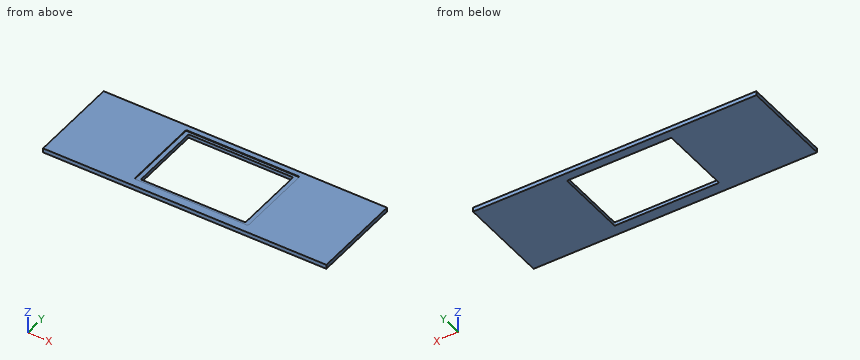
```python
from build123d import *

# Parameters (mm, degrees)
F0_W     = 1990
F0_H     = 645
F1_DEPTH = 30
F3_DEPTH = 5


with BuildPart() as f1:
    # F0 (on Top) → F1 (new body)
    with BuildSketch(Plane.XY):
        with Locations((-995, 322.5)):
            Rectangle(F0_W, F0_H)
        with BuildLine():
            ThreePointArc((-1353.5, 579), (-1351.742641, 583.242641), (-1347.5, 585))
            Line((-1347.5, 585), (-625.5, 585))
            ThreePointArc((-625.5, 585), (-621.257359, 583.242641), (-619.5, 579))
            Line((-619.5, 579), (-619.5, 83))
            ThreePointArc((-619.5, 83), (-621.257359, 78.757359), (-625.5, 77))
            Line((-625.5, 77), (-1347.5, 77))
            ThreePointArc((-1347.5, 77), (-1351.742641, 78.757359), (-1353.5, 83))
            Line((-1353.5, 83), (-1353.5, 579))
        make_face(mode=Mode.SUBTRACT)
    extrude(amount=F1_DEPTH)

    # F2 (on face) → F3 (cut)
    with BuildSketch(Plane.XY.offset(30)):
        with BuildLine():
            Line((-587.5, 65), (-587.5, 597))
            ThreePointArc((-587.5, 597), (-590.136039, 603.363961), (-596.5, 606))
            Line((-596.5, 606), (-1376.5, 606))
            ThreePointArc((-1376.5, 606), (-1382.863961, 603.363961), (-1385.5, 597))
            Line((-1385.5, 597), (-1385.5, 65))
            ThreePointArc((-1385.5, 65), (-1382.863961, 58.636039), (-1376.5, 56))
            Line((-1376.5, 56), (-596.5, 56))
            ThreePointArc((-596.5, 56), (-590.136039, 58.636039), (-587.5, 65))
        make_face()
        with BuildLine():
            Line((-625.5, 77), (-1347.5, 77))
            ThreePointArc((-1347.5, 77), (-1351.742641, 78.757359), (-1353.5, 83))
            Line((-1353.5, 83), (-1353.5, 579))
            ThreePointArc((-1353.5, 579), (-1351.742641, 583.242641), (-1347.5, 585))
            Line((-1347.5, 585), (-625.5, 585))
            ThreePointArc((-625.5, 585), (-621.257359, 583.242641), (-619.5, 579))
            Line((-619.5, 579), (-619.5, 83))
            ThreePointArc((-619.5, 83), (-621.257359, 78.757359), (-625.5, 77))
        make_face(mode=Mode.SUBTRACT)
    extrude(amount=-F3_DEPTH, mode=Mode.SUBTRACT)


solid = f1.part
```
Model file for the job. Use its own axes, mm. Coordinates: 2 decimals unless noted, no trailing zeros. Write each loop counter-clockwise with the first axis right and the second up, starting at its lowest first coordinate (ties: lowest second). Pieces come first, ordered by that corner, then holes. Notation, with made-up numbers: (-14, -16.5) - (-9, -16.5) arc R15 ccw to (-9, 9.5) - close; hole circle Ø7 at (73, -4.5). An arc over 180 degrees is marked (long way). Use a Markdown table: item, result. Add a question column.
Item 1: Band-saw the part on A-A, the plane y = 250.5. Write the cut outline in (x, z), and give its area (3 significant figures).
Item 2: Drill centre lines: line 1 along X through (y, z) = (399.5, 20.5); line 2 along X through (y, z) = (522, 27.5); line 3 along Y through (x, z) = (-725.5, 1.5). Where is each one in solid material? Low to high.
Item 3: Band-saw the part on C-C, the plane x = -772.5. Write the cut outline in (y, z), and give its area (3 significant figures).
Item 4: Band-saw the part on B-B, the plane z = 15.25. Write the cut outline in (x, y), and give its area (3 significant figures).
A:
| question | item | result |
|---|---|---|
| 1 | outline | (-1990, 0) - (-1353.5, 0) - (-1353.5, 25) - (-1385.5, 25) - (-1385.5, 30) - (-1990, 30) - close; (-619.5, 0) - (0, 0) - (0, 30) - (-587.5, 30) - (-587.5, 25) - (-619.5, 25) - close |
| 1 | area | 37,400 mm² |
| 2 | line 1 | x = -1990 to -1353.5, -619.5 to 0 |
| 2 | line 2 | x = -1990 to -1385.5, -587.5 to 0 |
| 2 | line 3 | y = 0 to 77, 585 to 645 |
| 3 | outline | (0, 0) - (77, 0) - (77, 25) - (56, 25) - (56, 30) - (0, 30) - close; (585, 0) - (645, 0) - (645, 30) - (606, 30) - (606, 25) - (585, 25) - close |
| 3 | area | 3,900 mm² |
| 4 | outline | (-1990, 0) - (0, 0) - (0, 645) - (-1990, 645) - close; hole (-1353.5, 83) arc R6 ccw to (-1347.5, 77) - (-625.5, 77) arc R6 ccw to (-619.5, 83) - (-619.5, 579) arc R6 ccw to (-625.5, 585) - (-1347.5, 585) arc R6 ccw to (-1353.5, 579) - close |
| 4 | area | 911,000 mm² |
